Could you check a few things on this model? Use its own coordinates, in mm. A direction names the side the tool comes from. Give positions to 0.01 mm unless a question says otherwise; leave off trailing zeros. Loops run counter-clockwise (first coordinate to the right, second up) from the corner with the lowest first, then second, coordinate; pieces in that order, holes last. Notation, with made-up numbers: M -21.75,-39.75 L 31.25,-39.75 A10 ccw 31.25,-26.75 Z; hole C -39.75,39 d6. An arc over 180 degrees is marked long. Answer in a Markdown table with one row per item. Add a question column.
```python
from build123d import *

# Parameters (mm, degrees)
SZKIC1_R                               = 20
DODANIE_WYCI_GNI_CIE1_DEPTH            = 50
DODANIE_WYCI_GNI_CIE4_DEPTH            = 40
SZKIC7_R                               = 10
WYTNIJ_WYCI_GNI_CIE1_DEPTH             = 40
WYTNIJ_WYCI_GNI_CIE1_DIRECTION_2_REACH = 99.268
ZAOKR_GLENIE1_R                        = 8
ZAOKR_GLENIE1_OF_LUSTRO2_R             = 8


with BuildPart() as part:
    # Szkic1 → Dodanie-wyciągnięcie1 (new body)
    with BuildSketch(Plane.XY):
        Circle(SZKIC1_R)
    dodanie_wyci_gni_cie1 = extrude(amount=DODANIE_WYCI_GNI_CIE1_DEPTH)

    # Szkic6 → Dodanie-wyciągnięcie4 (add)
    with BuildSketch(Plane.XY.offset(50)):
        with BuildLine():
            Line((-16, 12), (-16, 11))
            Line((-16, 11), (16, 11))
            Line((16, 11), (16, 12))
            ThreePointArc((16, 12), (0, 20), (-16, 12))
        make_face()
        with BuildLine():
            Line((16, -11), (16, -12))
            ThreePointArc((16, -12), (0, -20), (-16, -12))
            Line((-16, -12), (-16, -11))
            Line((-16, -11), (16, -11))
        make_face()
    dodanie_wyci_gni_cie4 = extrude(amount=DODANIE_WYCI_GNI_CIE4_DEPTH)

    # Szkic7 → Wytnij-wyciągnięcie1 (cut)
    with BuildSketch(Plane(origin=(0, -11, 0), x_dir=(1, 0, 0), z_dir=(0, 1, 0))):
        with Locations(Location((0, -75, 0), (0, 0, 270))):
            Circle(SZKIC7_R)
    wytnij_wyci_gni_cie1 = extrude(amount=WYTNIJ_WYCI_GNI_CIE1_DEPTH, mode=Mode.SUBTRACT)

    # Szkic7 → Wytnij-wyciągnięcie1 direction 2 (cut, up to next)
    with BuildSketch(Plane(origin=(0, -11, 0), x_dir=(1, 0, 0), z_dir=(0, 1, 0)), mode=Mode.PRIVATE) as wytnij_wyci_gni_cie1_direction_2_sk1:
        with Locations(Location((0, -75, 0), (0, 0, 270))):
            Circle(SZKIC7_R)
    wytnij_wyci_gni_cie1_direction_2_tool1 = extrude(wytnij_wyci_gni_cie1_direction_2_sk1.sketch, amount=-WYTNIJ_WYCI_GNI_CIE1_DIRECTION_2_REACH, mode=Mode.PRIVATE) & part.part
    wytnij_wyci_gni_cie1_direction_2 = wytnij_wyci_gni_cie1_direction_2_tool1.solids().sort_by_distance((0, -11, 75))[0]
    add(wytnij_wyci_gni_cie1_direction_2, mode=Mode.SUBTRACT)

    # Zaokrąglenie1
    zaokr_glenie1_edges = [part.edges().sort_by_distance(p)[0] for p in [
        (0, -11, 50),
        (0, 11, 50),
    ]]
    fillet(zaokr_glenie1_edges, radius=ZAOKR_GLENIE1_R)

    # Lustro2: Dodanie-wyciągnięcie1, Dodanie-wyciągnięcie4, Wytnij-wyciągnięcie1, Wytnij-wyciągnięcie1 direction 2 across plane
    add(dodanie_wyci_gni_cie1.mirror(Plane.XY))
    add(dodanie_wyci_gni_cie4.mirror(Plane.XY))
    add(wytnij_wyci_gni_cie1.mirror(Plane.XY), mode=Mode.SUBTRACT)
    add(wytnij_wyci_gni_cie1_direction_2.mirror(Plane.XY), mode=Mode.SUBTRACT)

    # Zaokrąglenie1 of Lustro2
    zaokr_glenie1_of_lustro2_edges = [part.edges().sort_by_distance(p)[0] for p in [
        (0, -11, -50),
        (0, 11, -50),
    ]]
    fillet(zaokr_glenie1_of_lustro2_edges, radius=ZAOKR_GLENIE1_OF_LUSTRO2_R)


solid = part.part
```
Item 1: For faces 4 (the face through (16, 11.15, 65.46)), 5 (the face through (-16, 11.2, 64)), 6 (the face through (-16, 11.2, -64)), 7 (the face through (0.224, -8.594, 52.281)), 8 (the face through (0.224, -8.594, -52.281)), which set-ups out of +Z, -Z, +X, -X, +Y, -Y let a thin tool reach every point of the face, with its end or its side?
Item 2: For P1, Ø4, axis at x = -9.5, z = 52.5, coming from the -Y side; P2, Ø10, axis at y = -6.5, z = -79.5, coming from the -X side; P3, Ø1.5, axis at x = 0.5, y = -6, coming from the +Z side; P4, Ø2.5, axis at y = 8, z = -64, coming from the +X side, each with a flat end and sliding along its axis, tell me the tip position at first contact or that it passes through.
Item 3: If we mould it in two halves opening along Y, with no side actions, what happens to faces 1 (the face through (-7, -11, 67)), 2 (the face through (-16, -11.2, 64)), 3 (the face through (-7, 11, -67))? For each: +Y half, -Y half, draft (parallel to the pull), parting line (faces both ways), or undercut.
Item 4: Suppose I cut it at D-D (y = -6.5). List the corners of the cut face in (x, z) for me.
Item 5: I need wall thicknesses on L1, parallel to Z at x = 0, y = -16.75; L2, parallel to Z at x = 8.5, y = 16; L3, parallel to Z at x = -8, y = -1.5. Which ranges of each line are inside material? Lowest first, please.
Item 6: Suppose I cut it at A-A (x = 0). Give the number of separate pieces and of enclosed holes in the cut face, then the cut area to 3 significant figures.
Item 7: Suppose I cut it at B-B (z = -75). List the corners of the cut face in (x, y) for me, then the cut area to 3 significant figures.
Item 8: Suppose I cut it at C-C (y = -16). List the corners of the cut face in (x, z) for me, then the cut area to 3 significant figures.
Values found:
| question | item | result |
|---|---|---|
| 1 | face 4 | +Z, +X, +Y, -Y |
| 1 | face 5 | +Z, -X, +Y, -Y |
| 1 | face 6 | -Z, -X, +Y, -Y |
| 1 | face 7 | +Z, +X, -X |
| 1 | face 8 | -Z, +X, -X |
| 2 | P1 | y = -18.54 |
| 2 | P2 | x = -16 |
| 2 | P3 | z = 50.93 |
| 2 | P4 | through |
| 3 | face 1 | undercut |
| 3 | face 2 | draft |
| 3 | face 3 | undercut |
| 4 | outline | M -18.91,-50 L -16,-50 L -16,-50.81 L 16,-50.81 L 16,-50 L 18.91,-50 L 18.91,50 L 16,50 L 16,50.81 L -16,50.81 L -16,50 L -18.91,50 Z |
| 5 | L1 | -90 to -85, -65 to 65, 85 to 90 |
| 5 | L2 | -90 to -80.27, -69.73 to 69.73, 80.27 to 90 |
| 5 | L3 | -50 to 50 |
| 6 | separate pieces | 5 |
| 6 | enclosed holes | 0 |
| 6 | area | 4,770 mm² |
| 7 | outline | M -16,-12 A20 ccw -10,-17.32 L -10,-11 L -16,-11 Z; M -16,11 L -10,11 L -10,17.32 A20 ccw -16,12 Z; M 10,-17.32 A20 ccw 16,-12 L 16,-11 L 10,-11 Z; M 10,11 L 16,11 L 16,12 A20 ccw 10,17.32 Z |
| 7 | area | 96.5 mm² |
| 8 | outline | M -12,-90 L 12,-90 L 12,90 L -12,90 Z; hole C 0,-75 d20; hole C 0,75 d20 |
| 8 | area | 3,690 mm² |
